from build123d import *

# Parameters (mm, degrees)
BOSS_EXTRUDE1_DEPTH = 3
BOSS_EXTRUDE2_START = 3
SKETCH1_3_R         = 1.45
BOSS_EXTRUDE2_DEPTH = 3


with BuildPart() as part:
    # Sketch1 → Boss-Extrude1 (new body)
    with BuildSketch(Plane(origin=(0, 0, 0), x_dir=(1, 0, 0), z_dir=(0, 1, 0))):
        with BuildLine():
            ThreePointArc((-0.961022379, 15.276470588), (-3.11550152, 9.263204593), (-6.019034903, 3.573684211))
            ThreePointArc((-6.019034903, 3.573684211), (0, -7), (6.019034903, 3.573684211))
            ThreePointArc((6.019034903, 3.573684211), (3.11550152, 9.263204593), (0.961022379, 15.276470588))
            ThreePointArc((0.961022379, 15.276470588), (0, 16), (-0.961022379, 15.276470588))
        make_face()
        with BuildLine():
            Line((-3.122498999, 2.5), (3.122498999, 2.5))
            ThreePointArc((3.122498999, 2.5), (0, -4), (-3.122498999, 2.5))
        make_face(mode=Mode.SUBTRACT)
    extrude(amount=-BOSS_EXTRUDE1_DEPTH)

    # Sketch1_3 → Boss-Extrude2 (add)
    with BuildSketch(Plane(origin=(0, 0, 0), x_dir=(1, 0, 0), z_dir=(0, 1, 0)).offset(BOSS_EXTRUDE2_START)):
        with BuildLine():
            ThreePointArc((-0.961022379, 15.276470588), (-3.11550152, 9.263204593), (-6.019034903, 3.573684211))
            ThreePointArc((-6.019034903, 3.573684211), (0, -7), (6.019034903, 3.573684211))
            ThreePointArc((6.019034903, 3.573684211), (3.11550152, 9.263204593), (0.961022379, 15.276470588))
            ThreePointArc((0.961022379, 15.276470588), (0, 16), (-0.961022379, 15.276470588))
        make_face()
        with Locations(Location((0, 0, 0), (0, 0, 270))):
            Circle(SKETCH1_3_R, mode=Mode.SUBTRACT)
    extrude(amount=-BOSS_EXTRUDE2_DEPTH)


solid = part.part
Read the model definition and answer for the solid it produces. Units are mm, in the model's axes. A direction names the side the tool comes from. Give positions to 0.01 mm unless a question says otherwise; leave off trailing zeros. Write each loop counter-clockwise with the first axis right and the second up, starting at its lowest first coordinate (ties: lowest second). Pieces come first, ordered by that corner, then holes. Notation, with made-up numbers: M -11.75,17 L 10.25,17 A7 cw 10.25,23 Z; hole C 28.25,4 d3. An arc over 180 degrees is marked long. One line per item, written item: value. Start each with the question number.
(1) Find section B-B (x = 0). Determine the outline of the cut face in (y, z), plus the area to 3 significant figures.
(2) Determine the mould class of faces 1 (the flat face through (0.8, 0, 1.4)), 2 (the flat face through (0, 3, -2)), 3 (the cylindrical face through (3.15, 0.04, -9.18)) for opening direction X: pulls with the +X half, pulls with the -X half, needs draft (parallel to the pull), parting line crosses it, or undercut.
(3) Find section D-D (x = -2). Determine the outline of the cut face in (y, z).
(4) Find section C-C (y = -1). Determine the outline of the cut face in (x, z), plus the area to 3 significant figures.
(5) A tool of negligible diameter and unlimited length cuts with its end or side. For faces 4 (the flat face through (0, -1, -2.5)), 5 (the cylindrical face through (-3.1, 0, -9.3)), from which of +Z, -Z, +X, -X, +Y, -Y can it reach the whole face along a straight path? Write none if from no direction.
(6) Flat-ended cylindrical pins translate along their axes: pin 1 Ø2.5 at (x, z) = (0, 0) entering from +Y; pin 2 Ø1.5 at (y, z) = (2, -9) entering from -X; pin 3 Ø1.5 at (y, z) = (1.5, 4.5) entering from -X. Find the tip coordinate at first contact, or state that the pin passes through.
(7) Find section A-A (z = 0). Determine the outline of the cut face in (x, y), plus the area to 3 significant figures.
(8) Find the intervals of material crossed by line 1 (X direction, y = -0.75, z = 0); line 2 (Y direction, x = 0.25, z = 2); line 3 (Z direction, x = -3.25, y = -1.9), in increasing order.
Results below:
1. outline: M -3,-16 L 3,-16 L 3,-1.45 L 0,-1.45 L 0,-2.5 L -3,-2.5 Z; M -3,4 L 0,4 L 0,1.45 L 3,1.45 L 3,7 L -3,7 Z
1. area: 110 mm^2
2. face 1: undercut
2. face 2: needs draft
2. face 3: pulls with the +X half
3. outline: M -3,-12.07 L 3,-12.07 L 3,6.71 L -3,6.71 L -3,3.46 L 0,3.46 L 0,-2.5 L -3,-2.5 Z
4. outline: M -6.02,-3.57 A50 cw -0.96,-15.28 A1 ccw 0.96,-15.28 A50 cw 6.02,-3.57 A7 ccw long Z; hole M -3.12,-2.5 L 3.12,-2.5 A4 ccw long Z
4. area: 157 mm^2
5. face 4: -Y
5. face 5: -Z, -X, +Y, -Y
6. pin 1: passes through
6. pin 2: stops at x = -3.57
6. pin 3: stops at x = -5.91
7. outline: M -7,-3 L -4,-3 L -4,0 L -1.45,0 L -1.45,3 L -7,3 Z; M 1.45,0 L 4,0 L 4,-3 L 7,-3 L 7,3 L 1.45,3 Z
7. area: 51.3 mm^2
8. line 1: x = -7 to -4, 4 to 7
8. line 2: y = 0 to 3
8. line 3: z = -8.95 to -2.33, 2.33 to 6.2
